Part model, mm, in its own coordinate system. A direction names the side the tool comes from. Round coordinates to 2 decimals unless told otherwise and drop trailing zeros. Loops run counter-clockwise (first coordinate to the right, second up) from the corner with the lowest first, then second, coordinate; pieces in that order, holes last. Notation, with made-up numbers: M 83.5,-39 L 119.5,-39 A15 cw 119.5,-16 Z; hole C 76,68 d6. An arc over 180 degrees is marked long. Put each result on its own line as item: value. Start each with the question number.
1) Slice it at D-D on z = 2. Give the cut face in (x, y).
2) Pull direction Z, two halves, no side cores. Call faces 6 (the cylindrical face through (-8.929, -2.2, 2.194)), 7 (the flat face through (-8, -1.5, 3)), 8 (the flat face through (-8, 4.83, -1)), 9 (the flat face through (-12.4, 2.5, -3.27)): +Z half, -Z half, draft (parallel to the pull), parting line (faces both ways), or undercut.
3) Probe line 1 along X through (y, z) = (-2.45, 3.3) (3 decimals); line 2 along X through (y, z) = (0.1, 4.05); line 3 along Z through (x, y) = (-12.5, 0.5). List the from-to ranges inside material, lowest first.
4) Slice it at B-B on y = 1.5. Give the cut face in (x, z), then the cut area to 3 significant figures.
5) Slice it at C-C on x = -11.25. Give the cut face in (y, z), then the cut area to 3 significant figures.
6) Drop flat-ended pins along their axis: pin 1 Ø3 at (x, z) = (-3.96, 4.05) entering from -Y; pin 2 Ø3 at (x, z) = (-4.5, 3) entering from +Y; pin 3 Ø2.5 at (x, y) = (-3.96, 0.86) entering from -Z. Give the stop position or say it passes through.
7) Slice it at A-A on y = -2. Give the cut face in (x, z) (3 decimals).
8) Which spindle directions (+Z, -Z, +X, -X, +Y, -Y) get a long thin tool onto all of the face, cutting with end or side? Do faces 1 (the flat face through (-8, 0, 4)), 2 (the flat face through (-12, 2.1, 4)), 3 (the flat face through (-8, -2, 6.6)), 4 (the cylindrical face through (-9.443, 0.536, -2.373)), 5 (the flat face through (-3.9, 2.5, -3.27)). Say none if no direction does.
```python
from build123d import *

# Parameters (mm, degrees)
BOSS_EXTRUDE1_DEPTH = 15.83
SKETCH2_R           = 2.45
BOSS_EXTRUDE2_DEPTH = 2.1
SHELL1_START        = -3.12
SHELL1_OUTLINE_W    = 12.83
SHELL1_OUTLINE_H    = 6.6
SHELL1_DEPTH        = 1.62
SHELL1_START_2      = -1.5
SHELL1_2_OUTLINE_R  = 0.95
SHELL1_2_DEPTH      = 2.1
SKETCH3_R           = 2.45
SKETCH3_R_2         = 1.47
SKETCH3_R_3         = 1.51
BOSS_EXTRUDE3_DEPTH = 1.77
SKETCH4_R           = 1.5
SKETCH4_R_2         = 0.66
BOSS_EXTRUDE4_DEPTH = 1.42


# Read off the part's stored shape, not the designer's step: Shell1
with BuildPart() as part:
    # Sketch1 → Boss-Extrude1 (new body)
    with BuildSketch(Plane(origin=(0, 0, 0), x_dir=(0, 0, -1), z_dir=(1, 0, 0))):
        Polygon((0, 0), (0, 4.83), (1.5, 4.83), (1.5, -3.12), (-8.1, -3.12), (-8.1, 0), align=None)
    extrude(amount=-BOSS_EXTRUDE1_DEPTH)

    # Sketch2 → Boss-Extrude2 (add)
    with BuildSketch(Plane(origin=(0, 0, 0), x_dir=(1, 0, 0), z_dir=(0, 1, 0))):
        with Locations(Location((-11.8725, -4.05, 0), (0, 0, 270))):
            Circle(SKETCH2_R)
        with Locations(Location((-3.9575, -4.05, 0), (0, 0, 270))):
            Circle(SKETCH2_R)
    extrude(amount=BOSS_EXTRUDE2_DEPTH)

    # Shell1 outline → Shell1 (cut)
    with BuildSketch(Plane(origin=(0, 0, 0), x_dir=(1, 0, 0), z_dir=(0, 1, 0)).offset(SHELL1_START)):
        with Locations((-7.915, -3.3)):
            Rectangle(SHELL1_OUTLINE_W, SHELL1_OUTLINE_H)
    extrude(amount=SHELL1_DEPTH, mode=Mode.SUBTRACT)

    # Shell1 2 outline → Shell1 2 (cut)
    with BuildSketch(Plane(origin=(0, 0, 0), x_dir=(1, 0, 0), z_dir=(0, 1, 0)).offset(SHELL1_START_2)):
        with Locations((-11.8725, -4.05)):
            Circle(SHELL1_2_OUTLINE_R)
        with Locations((-3.9575, -4.05)):
            Circle(SHELL1_2_OUTLINE_R)
    extrude(amount=SHELL1_2_DEPTH, mode=Mode.SUBTRACT)

    # Sketch3 → Boss-Extrude3 (add)
    # profile 1 of 2: a face of its own
    with BuildSketch(Plane(origin=(0, 0, -1.5), x_dir=(-1, 0, 0), z_dir=(0, 0, -1))):
        with Locations(Location((3.9575, 0.855, 0), (0, 0, 90))):
            Circle(SKETCH3_R)
        with Locations(Location((3.9575, 0.855, 0), (0, 0, 90))):
            Circle(SKETCH3_R_2, mode=Mode.SUBTRACT)
    # profile 2 of 2: a face of its own
    with BuildSketch(Plane(origin=(0, 0, -1.5), x_dir=(-1, 0, 0), z_dir=(0, 0, -1))):
        with Locations(Location((11.8725, 0.855, 0), (0, 0, 90))):
            Circle(SKETCH3_R)
        with Locations(Location((11.8725, 0.855, 0), (0, 0, 90))):
            Circle(SKETCH3_R_3, mode=Mode.SUBTRACT)
    extrude(amount=BOSS_EXTRUDE3_DEPTH)

    # Sketch4 → Boss-Extrude4 (add)
    with BuildSketch(Plane.XZ.offset(1.5)):
        with Locations(Location((-7.915, 3.3, 0), (0, 0, 90))):
            Circle(SKETCH4_R)
        with Locations(Location((-7.915, 3.3, 0), (0, 0, 270))):
            Circle(SKETCH4_R_2, mode=Mode.SUBTRACT)
    extrude(amount=BOSS_EXTRUDE4_DEPTH)


solid = part.part
```
Recorded:
1. outline: M -15.83,-3.12 L -14.33,-3.12 L -14.33,-1.5 L -8.66,-1.5 L -8.66,-2.92 L -7.17,-2.92 L -7.17,-1.5 L -1.5,-1.5 L -1.5,-3.12 L 0,-3.12 L 0,0 L -2.62,0 L -2.62,2.1 L -5.3,2.1 L -5.3,0 L -10.53,0 L -10.53,2.1 L -13.21,2.1 L -13.21,0 L -15.83,0 Z
2. face 6: undercut
2. face 7: undercut
2. face 8: draft
2. face 9: -Z half
3. line 1: x = -15.83 to -14.33, -9.415 to -8.575, -7.255 to -6.415, -1.5 to 0
3. line 2: x = -14.32 to -12.82, -10.92 to -9.42, -6.41 to -4.91, -3.01 to -1.51
3. line 3: z = -1.5 to 0, 1.68 to 3.34, 4.76 to 6.42
4. outline: M -15.83,-1.5 L -14.24,-1.5 L -14.24,-3.27 L -13.24,-3.27 L -13.24,-1.5 L -10.51,-1.5 L -10.51,-3.27 L -9.51,-3.27 L -9.51,-1.5 L -6.32,-1.5 L -6.32,-3.27 L -5.28,-3.27 L -5.28,-1.5 L -2.64,-1.5 L -2.64,-3.27 L -1.59,-3.27 L -1.59,-1.5 L 0,-1.5 L 0,0 L -15.83,0 Z; C -11.87,4.05 d4.9; C -3.96,4.05 d4.9
4. area: 68.7 mm2
5. outline: M -3.12,-1.5 L -1.51,-1.5 L -1.51,-3.27 L -0.52,-3.27 L -0.52,-1.5 L 2.23,-1.5 L 2.23,-3.27 L 3.22,-3.27 L 3.22,-1.5 L 4.83,-1.5 L 4.83,0 L 0,0 L 0,1.68 L 2.1,1.68 L 2.1,6.42 L 0,6.42 L 0,8.1 L -3.12,8.1 L -3.12,6.6 L -1.5,6.6 L -1.5,4.77 L 0.6,4.77 L 0.6,3.33 L -1.5,3.33 L -1.5,0 L -3.12,0 Z
5. area: 37.0 mm2
6. pin 1: stops at y = -1.5
6. pin 2: stops at y = 2.1
6. pin 3: stops at z = -1.5
7. outline: M -15.83,-1.5 L 0,-1.5 L 0,8.1 L -15.83,8.1 Z; C -7.915,3.3 d3; hole M -14.33,0 L -1.5,0 L -1.5,6.6 L -14.33,6.6 Z; hole C -7.915,3.3 d1.32
8. face 1: +Y
8. face 2: +Z, +X, -X, +Y
8. face 3: -Y
8. face 4: -Z
8. face 5: -Z, +X, -X, +Y, -Y
